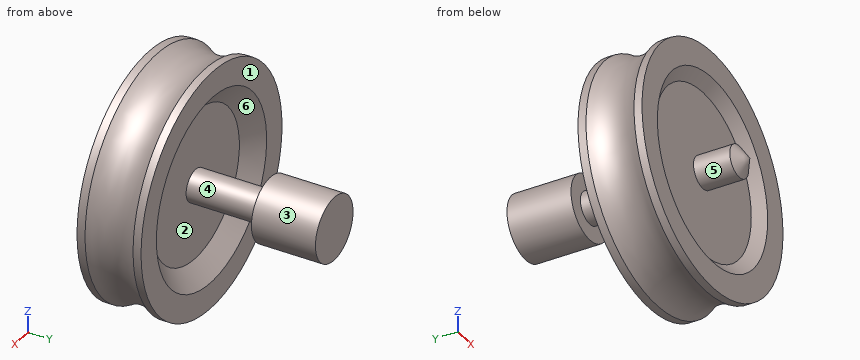
Autodesk Inventor part; units mm, degrees
ref_plane "YZ Plane" through (0, 0, 0) normal (1, 0, 0) x (0, 1, 0)
ref_plane "XZ Plane" through (0, 0, 0) normal (0, 1, 0) x (-1, 0, 0)
ref_plane "XY Plane" through (0, 0, 0) normal (0, 0, 1) x (1, 0, 0)
sketch "Sketch1" plane through (0, 0, 0) normal (0, 0, 1) x (1, 0, 0)
  line L0 (0, 0) -> (0, 21.1667)
  line L1 (0, 0) -> (0, -10.5833)
  line L2 (0, 21.1667) -> (0, 33.8667)
  line L3 (6.35, 21.1667) -> (6.35, 33.8667)
  line L4 (6.35, 33.8667) -> (0, 33.8667)
  line L5 (3.175, 12.7991) -> (0, 12.7991) construction
  line L6 (6.35, 21.1667) -> (3.175, 21.1667)
  line L7 (3.175, 21.1667) -> (0, 21.1667) construction
  line L8 (0, 0) -> (3.175, 0) construction
  line L9 (3.175, 0) -> (17.91, 0) construction
  line L10 (23.8125, 7.9375) -> (23.8125, 9.525)
  line L11 (14.8167, 6.35) -> (3.175, 6.35)
  line L12 (18.6267, 9.525) -> (23.8125, 9.525)
  line L13 (0, -10.5833) -> (3.175, -8.4667)
  line L14 (3.175, -8.4667) -> (3.175, 0)
  line L15 (14.8167, 6.35) -> (18.6267, 9.525)
  line L16 (3.175, 21.1667) -> (3.175, 6.35)
  line L17 (1.0583, 6.35) -> (3.175, 6.35) construction
  line L18 (1.0583, 6.35) -> (1.0583, 3.175) construction
  line L19 (1.0583, 3.175) -> (5.214, 3.175) construction
  line L20 (23.8125, -1.5875) -> (23.8125, -3.175)
  line L21 (14.8167, 0) -> (3.175, 0)
  line L22 (18.6267, -3.175) -> (23.8125, -3.175)
  line L23 (14.8167, 0) -> (18.6267, -3.175)
  line L24 (3.175, 0) -> (3.175, 0)
  arc A0 (23.8125, 7.9375) -> (23.8125, -1.5875) centre (30.8127, 3.175) ccw
  line L25 (23.8125, -3.175) -> (23.495, -3.175)
  dimension "d5" = 44.45
  dimension "d6" = 12.7
  dimension "d7" = 6.35
  dimension "d12" = 2.1167
  dimension "d13" = 3.175
  dimension "d15" = 8.4667
  dimension "d18" = 1.5875
  dimension "d20" = 3.175
  dimension "d21" = 3.81
  dimension "d26" = 23.8125
  dimension "d30" = 11.6417
  dimension "d31" = 3.175
  dimension "d32" = 2.1167
  dimension "d33" = 8.4667
  dimension "d34" = 3.175
  dimension "d36" = 0.3175
revolve "Revolution1" add sketch "Sketch1" angle 360 about axis through (0, 21.1667, 0) along (0, -1, 0)
move faces "Move1" translate (0, -1.27, 0) faces at (10.7618, 0, -1.4352)
properties part number "Top Spoolish"
For this review, take the finished solid that the model builds, in its own axes (mm). Face numbers are marked on the shaded views. A direction names the side the tool comes from. Give positions to 0.01 mm unless a question says otherwise; leave off trailing zeros. Order: outer loops, then holes, each group sorted by start corner. A loop starts at its lowest first (then second) coordinate and runs counter-clockwise, first axis right, second up.
1) The part is to be moulded in two halves that separate along X. For the marked faces 1, 2 and 3, say which applies: released by +X, released by -X, zero draft, split by the parting line, or undercut.
2) Wall thickness on line 1 (Y direction, x = 13, z = -15) (3 decimals); line 2 (Y direction, x = 8.5, z = -7.5); line 3 (Y direction, x = -12, z = -19.5) (3 decimals): over which ranges is each line inside the solid? List them lowest first.
3) For the marked faces 4, 5 and 6, list the 3-axis set-ups (+Z, -Z, +X, -X, +Y, -Y) from which the entire face can be reached by the end or side of a thin tool; tool diameter is ignored.
4) Take a section at A-A (y = 12). Give the boundary of the cut face in (x, z) (3 decimals), then the cut area to 3 significant figures.
5) Take a section at B-B (y = 25.5). Give the boundary of the cut face in (x, z), then the cut area to 3 significant figures.
6) Insertion check: pin 1 (1 mm diameter, centred on x = 2.5, y = 23, fed in from +Z); pin 2 (5 mm diameter, centred on x = 13, y = -0.5, fed in from -Z); pin 3 (5 mm diameter, centred on x = -5.5, y = 29, fed in from +Z); pin 4 (10 mm diameter, centred on x = 0.5, z = -3, fed in from -Y). Each pin has a flat end and moves straight along its axis. Give the tip position at first contact, or say it passes through.
Derived:
1. face 1: zero draft
1. face 2: undercut
1. face 3: split by the parting line
2. line 1: y = -3.175 to 9.525
2. line 2: y = -1.27 to 6.35
2. line 3: y = -3.175 to 0.172, 6.178 to 9.525
3. face 4: none
3. face 5: -Y
3. face 6: +Y
4. outline: circle Ø6.35 at (0, 0)
4. area: 31.7 mm2
5. outline: circle Ø12.7 at (0, 0)
5. area: 127 mm2
6. pin 1: stops at z = 6.03
6. pin 2: stops at z = -21.25
6. pin 3: stops at z = 5.6
6. pin 4: stops at y = -10.58
